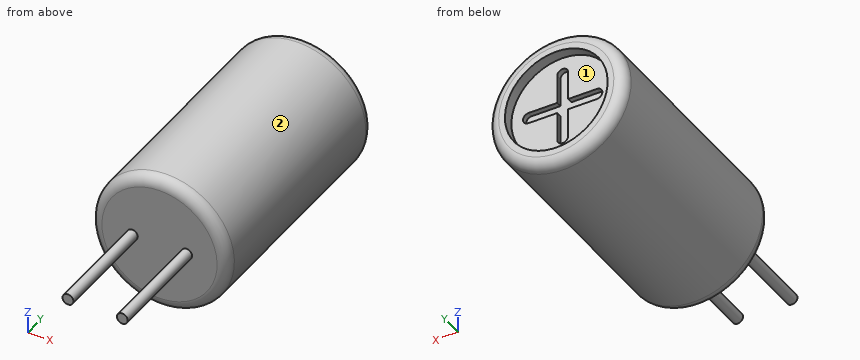
```python
from build123d import *

# Parameters (mm, degrees)
SKETCH_2_R          = 3.15
EXTRUDE_1_DEPTH     = 11.2
FILLET_1_R          = 0.5
SKETCH_3_R          = 0.25
EXTRUDE_2_DEPTH     = 5
SKETCH_5_R          = 2.3625
CUT_EXTRUDE_1_DEPTH = 1
EXTRUDE_START       = 0.5
SKETCH_6_R          = 2.3625
EXTRUDE_3_DEPTH     = 0.5
CUT_EXTRUDE_2_DEPTH = 0.25
CUT_EXTRUDE_3_DEPTH = 0.25


with BuildPart() as part:
    # 草图2 → 凸台-拉伸1 (new body)
    with BuildSketch(Plane(origin=(0, 0, 0), x_dir=(1, 0, 0), z_dir=(0, 1, 0))):
        with Locations(Location((0, 0, 0), (0, 0, 270))):
            Circle(SKETCH_2_R)
    extrude(amount=EXTRUDE_1_DEPTH)

    # 圆角1
    fillet_1_edges = [part.edges().sort_by_distance(p)[0] for p in [
        (0, 0, -3.15),
        (0, 11.2, -3.15),
    ]]
    fillet(fillet_1_edges, radius=FILLET_1_R)

    # 草图3 → 凸台-拉伸2 (add)
    with BuildSketch(Plane.XZ):
        with Locations(Location((-1.25, 0, 0), (0, 0, 90))):
            Circle(SKETCH_3_R)
        with Locations(Location((1.25, 0, 0), (0, 0, 90))):
            Circle(SKETCH_3_R)
    extrude(amount=EXTRUDE_2_DEPTH)

    # 草图5 → 切除-拉伸1 (cut)
    with BuildSketch(Plane(origin=(0, 11.2, 0), x_dir=(1, 0, 0), z_dir=(0, 1, 0))):
        with Locations(Location((0, 0, 0), (0, 0, 270))):
            Circle(SKETCH_5_R)
    extrude(amount=-CUT_EXTRUDE_1_DEPTH, mode=Mode.SUBTRACT)

    # 草图6 → 凸台-拉伸3 (add)
    with BuildSketch(Plane(origin=(0, 10.2, 0), x_dir=(1, 0, 0), z_dir=(0, 1, 0)).offset(EXTRUDE_START)):
        with Locations(Location((0, 0, 0), (0, 0, 270))):
            Circle(SKETCH_6_R)
    extrude(amount=-EXTRUDE_3_DEPTH)

    # 草图7 → 切除-拉伸2 (cut)
    with BuildSketch(Plane(origin=(0, 10.7, 0), x_dir=(1, 0, 0), z_dir=(0, 1, 0))):
        with BuildLine():
            Line((-1.575, 0.25), (1.575, 0.25))
            ThreePointArc((1.575, 0.25), (1.825, 0), (1.575, -0.25))
            Line((1.575, -0.25), (-1.575, -0.25))
            ThreePointArc((-1.575, -0.25), (-1.825, 0), (-1.575, 0.25))
        make_face()
    extrude(amount=-CUT_EXTRUDE_2_DEPTH, mode=Mode.SUBTRACT)

    # 草图8 → 切除-拉伸3 (cut)
    with BuildSketch(Plane(origin=(0, 10.7, 0), x_dir=(1, 0, 0), z_dir=(0, 1, 0))):
        with BuildLine():
            Line((-0.25, -1.575), (-0.25, 1.575))
            ThreePointArc((-0.25, 1.575), (0, 1.825), (0.25, 1.575))
            Line((0.25, 1.575), (0.25, -1.575))
            ThreePointArc((0.25, -1.575), (0, -1.825), (-0.25, -1.575))
        make_face()
    extrude(amount=-CUT_EXTRUDE_3_DEPTH, mode=Mode.SUBTRACT)


solid = part.part
```
The model under review builds one solid part; all positions refer to its coordinate system, in mm. Face numbers are marked on the shaded views. Round coordinates to 2 decimals unless told otherwise and drop trailing zeros. Write each loop counter-clockwise with the first axis right and the second up, starting at its lowest first coordinate (ties: lowest second). Pieces come first, ordered by that corner, then holes. Notation, with made-up numbers: (78.5, -40) - (127.5, -40) arc R14 cw to (127.5, -21) - close; hole circle Ø3 at (-2.5, 55.5). An arc over 180 degrees is marked (long way). Answer as CSV lines item,"result". Start each with the question number.
(1) To check wall thickness, follow line 1 (Y direction, x = 1.25, z = -1); line 2 (X direction, y = 11, z = 0); line 3 (X direction, y = 10.8, z = 0). State the ranges of each line that lie inside material, in increasing order.
(2) We need section C-C on y = -3. State the section outline as (x, z) points.
(3) Draft analysis for pull direction X (two halves, no side actions). For the marked faces 1 and 2, state which applies: pulls with the +X half, pulls with the -X half, needs draft (parallel to the pull), parting line crosses it, or undercut.
(4) We need section D-D on y = 6.25. State the section outline as (x, z) points.
(5) For pin 1 Ø1.5 at (x, z) = (-0.5, 0) entering from +Y; pin 2 Ø3 at (x, z) = (0, -2.5) entering from -Y, all flat-tipped, find the tip position at first contact; note any pin that passes through.
Worked answers:
1,line 1,"0 to 10.7"
1,line 2,"-3.05 to -2.36, 2.36 to 3.05"
1,line 3,"-3.14 to -2.36, 2.36 to 3.14"
2,outline,"circle Ø0.5 at (-1.25, 0); circle Ø0.5 at (1.25, 0)"
3,face 1,"undercut"
3,face 2,"parting line crosses it"
4,outline,"circle Ø6.3 at (0, 0)"
5,pin 1,"y = 10.7"
5,pin 2,"y = 0"
